For this review, use the dimensioned drawing (mm, ordinates from the lowest corner) and the shaded views. A direction names the side the tool comes from. Coordinates: 2 decimals unless noted, no trailing zeros. Order: outer loops, then holes, each group sorted by start corner. A loop starts at its lowest first (then second) coordinate and runs counter-clockwise, first axis right, second up. Notation, with made-up numbers: M 6,68 L 33,68 A31 ccw 33,99 Z; hole C -32,8 d4. An arc over 180 degrees is marked long. Answer in a Markdown table with one row per item.
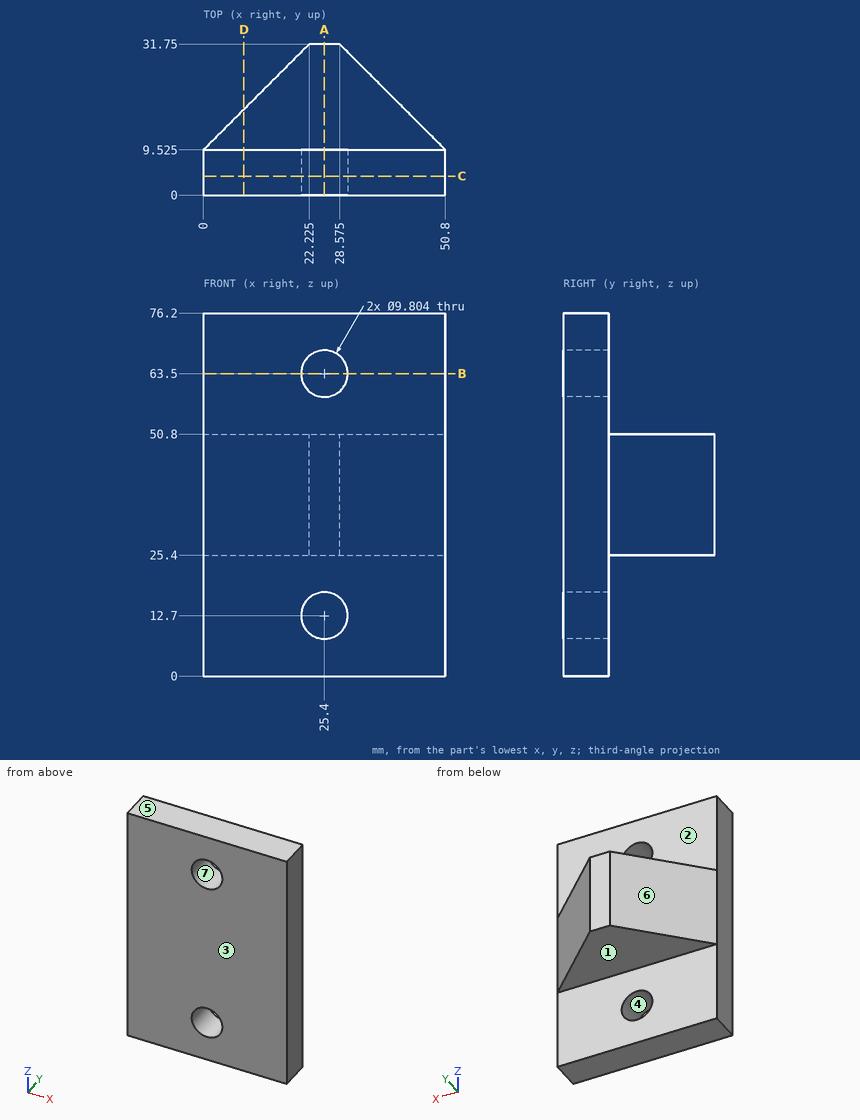
(1) Take a section at C-C (y = 4). Write out the cut boundary in (x, z) (1 decimal), then the cut area to 3 significant figures.
Report:
| item | result |
|---|---|
| outline | M 0,0 L 50.8,0 L 50.8,76.2 L 0,76.2 Z; hole C 25.4,12.7 d9.8; hole C 25.4,63.5 d9.8 |
| area | 3,720 mm^2 |
(2) Machinability: for the marked faces 1, 2 and 3, which of the approach directions +Z, -Z, +X, -X, +Y, -Y give a long, thin tool a straight path to every point of the face, cutting with its end or side? Answer none if there is none.
Report:
| item | result |
|---|---|
| face 1 | -Z, +X, -X, +Y |
| face 2 | +Z, +X, -X, +Y |
| face 3 | +Z, -Z, +X, -X, -Y |
(3) Take a section at A-A (x = 25.4). State how many separate pieces and enclosed holes the cut face has, then the cut area to 3 significant figures.
Report:
| item | result |
|---|---|
| separate pieces | 3 |
| enclosed holes | 0 |
| area | 1,100 mm^2 |
(4) To check wall thickness, follow line 1 (Z direction, x = 25.4, y = 7.25); line 2 (Y direction, x = 6.5, z = 8.5) (1 decimal); line 3 (Z direction, x = 29, y = 19). State the ranges of each line that lie inside material, in increasing order. Write a range as [from, to].
Report:
| item | result |
|---|---|
| line 1 | [0, 7.8], [17.6, 58.6], [68.4, 76.2] |
| line 2 | [0, 9.5] |
| line 3 | [25.4, 50.8] |
(5) Insertion check: P1, Ø6, axis at x = 35, y = 26, coming from the -Z side; P2, Ø7.5, axis at x = 30, z = 59.5, coming from the +Y side (3 decimals); P3, Ø12, axis at y = 19.5, z = 47.5, coming from the -X side (1 decimal). Each pin has a flat end and moves straight along its axis. Give the tip position at first contact, or say it passes through.
Report:
| item | result |
|---|---|
| P1 | z = 25.4 |
| P2 | y = 9.525 |
| P3 | x = 4 |
(6) Take a section at D-D (x = 8.5). Write out the cut boundary in (y, z) (1 decimal).
Report:
| item | result |
|---|---|
| outline | M 0,0 L 9.5,0 L 9.5,25.4 L 18,25.4 L 18,50.8 L 9.5,50.8 L 9.5,76.2 L 0,76.2 Z |
(7) Take a section at B-B (z = 63.5). Write out the cut boundary in (x, y) (1 decimal).
Report:
| item | result |
|---|---|
| outline | M 0,0 L 20.5,0 L 20.5,9.5 L 0,9.5 Z; M 30.3,0 L 50.8,0 L 50.8,9.5 L 30.3,9.5 Z |
(8) The part is to be moulded in two halves that separate along X. For the marked faces 4, 5, 6 and 7, say which applies: +X half, -X half, draft (parallel to the pull), parting line (faces both ways), or undercut.
Report:
| item | result |
|---|---|
| face 4 | undercut |
| face 5 | draft |
| face 6 | -X half |
| face 7 | undercut |
